Can you work these out from the model? Positions are in its coordinate system, mm. A direction names the side the tool comes from. Give positions to 0.01 mm unless a question says otherwise; leave off trailing zeros. Write each loop counter-clockwise with the first axis right and the second up, starting at its lowest first coordinate (ties: lowest second). Pieces come first, ordered by that corner, then holes.
from build123d import *

# Parameters (mm, degrees)
F0_W     = 2.7374038473
F0_H     = 4.5464726281
F1_DEPTH = 3


with BuildPart() as f1:
    # F0 (on Front) → F1 (new body)
    with BuildSketch(Plane.XZ):
        with BuildLine():
            Line((-13.9879264009, 8.4983842463), (-10.7078288449, 8.4983842463))
            ThreePointArc((-10.7078288449, 8.4983842463), (-12.3096819162, -5.9457433928), (0, -13.6704108706))
            Line((0, -13.6704108706), (29.832560569, -13.6704108706))
            ThreePointArc((29.832560569, -13.6704108706), (41.0439649972, -7.8220549805), (42.6626390029, 4.7190275219))
            ThreePointArc((42.6626390029, 4.7190275219), (52.7277631814, 0.6811115523), (57.2114773095, -9.193492122))
            Line((57.2114773095, -9.193492122), (57.2114773095, 27.5829305145))
            ThreePointArc((57.2114773095, 27.5829305145), (52.7277631814, 17.7083268402), (42.6626390029, 13.6704108706))
            Line((42.6626390029, 13.6704108706), (29.832560569, 13.6704108706))
            Line((29.832560569, 13.6704108706), (0, 13.6704108706))
            Line((0, 13.6704108706), (-14.4307379611, 13.6704108706))
            Line((-14.4307379611, 13.6704108706), (-14.8297163701, 14.5122008398))
            Line((-14.8297163701, 14.5122008398), (-15.268201828, 14.5122008398))
            ThreePointArc((-15.268201828, 14.5122008398), (-15.9753086092, 14.219307621), (-16.268201828, 13.5122008398))
            Line((-16.268201828, 13.5122008398), (-16.268201828, 9.0994058373))
            ThreePointArc((-16.268201828, 9.0994058373), (-15.9753086092, 8.3922990562), (-15.268201828, 8.0994058373))
            Line((-15.268201828, 8.0994058373), (-14.8297163701, 8.0994058373))
            Line((-14.8297163701, 8.0994058373), (-13.9879264009, 8.4983842463))
        make_face()
        with Locations((-10.5523099191, -3.12910098)):
            Rectangle(F0_W, F0_H, mode=Mode.SUBTRACT)
        Polygon((9.3416453156, -8.6632125312), (7.1077647943, -8.6632125312), (4.7967138551, -2.7617063542), (-2.6400774802, -2.7617063542), (-4.9226972128, -8.6632125312), (-7.1078385226, -8.6632125312), (0.2274127889, 9.9714126168), (2.0429484125, 9.9714126168), align=None, mode=Mode.SUBTRACT)
        with Locations((-10.5523099191, 3.0826488801)):
            Rectangle(F0_W, F0_H, mode=Mode.SUBTRACT)
        with BuildLine():
            Line((11.8923307107, -8.6632125312), (11.8923307107, 9.8942421988))
            Line((11.8923307107, 9.8942421988), (17.1358575342, 9.8942421988))
            add(Edge.make_bspline(
                [(17.1358575342, 9.8942421988), (20.8278527957, 9.8942421988), (22.4788935809, 8.7894867411)],
                knots=[0, 0, 0, 1, 1, 1], degree=2))
            add(Edge.make_bspline(
                [(22.4788935809, 8.7894867411), (24.1299343662, 7.6847312833), (24.1299343662, 5.300571527)],
                knots=[0, 0, 0, 1, 1, 1], degree=2))
            add(Edge.make_bspline(
                [(24.1299343662, 5.300571527), (24.1299343662, 3.6474999413), (23.2099817515, 2.5752372911)],
                knots=[0, 0, 0, 1, 1, 1], degree=2))
            add(Edge.make_bspline(
                [(23.2099817515, 2.5752372911), (22.2900291369, 1.5029746409), (20.5232327246, 1.1861697669)],
                knots=[0, 0, 0, 1, 1, 1], degree=2))
            Line((20.5232327246, 1.1861697669), (20.5232327246, 1.0602601376))
            add(Edge.make_bspline(
                [(20.5232327246, 1.0602601376), (24.7513593112, 0.3372951689), (24.7513593112, -3.3831312992)],
                knots=[0, 0, 0, 1, 1, 1], degree=2))
            add(Edge.make_bspline(
                [(24.7513593112, -3.3831312992), (24.7513593112, -5.8688310792), (23.0698565188, -7.2660218052)],
                knots=[0, 0, 0, 1, 1, 1], degree=2))
            add(Edge.make_bspline(
                [(23.0698565188, -7.2660218052), (21.3883537265, -8.6632125312), (18.3665226214, -8.6632125312)],
                knots=[0, 0, 0, 1, 1, 1], degree=2))
            Line((18.3665226214, -8.6632125312), (11.8923307107, -8.6632125312))
        make_face(mode=Mode.SUBTRACT)
        with BuildLine():
            add(Edge.make_bspline(
                [(38.1099648282, -0.6293658567), (39.2065970841, -1.8234765353), (39.2065970841, -3.7243057788)],
                knots=[0, 0, 0, 1, 1, 1], degree=2))
            add(Edge.make_bspline(
                [(39.2065970841, -3.7243057788), (39.2065970841, -6.1734511503), (37.4296466694, -7.5462722706)],
                knots=[0, 0, 0, 1, 1, 1], degree=2))
            add(Edge.make_bspline(
                [(37.4296466694, -7.5462722706), (35.6526962548, -8.919093391), (32.606495544, -8.919093391)],
                knots=[0, 0, 0, 1, 1, 1], degree=2))
            add(Edge.make_bspline(
                [(32.606495544, -8.919093391), (29.3084755745, -8.919093391), (27.5294943594, -8.0661571919)],
                knots=[0, 0, 0, 1, 1, 1], degree=2))
            Line((27.5294943594, -8.0661571919), (27.5294943594, -5.9866175067))
            add(Edge.make_bspline(
                [(27.5294943594, -5.9866175067), (28.6748658267, -6.4658864185), (30.0192557403, -6.7461368839)],
                knots=[0, 0, 0, 1, 1, 1], degree=2))
            add(Edge.make_bspline(
                [(30.0192557403, -6.7461368839), (31.363645654, -7.0263873493), (32.683665962, -7.0263873493)],
                knots=[0, 0, 0, 1, 1, 1], degree=2))
            add(Edge.make_bspline(
                [(32.683665962, -7.0263873493), (34.8403760653, -7.0263873493), (35.9329467202, -6.2079747584)],
                knots=[0, 0, 0, 1, 1, 1], degree=2))
            add(Edge.make_bspline(
                [(35.9329467202, -6.2079747584), (37.0255173751, -5.3895621674), (37.0255173751, -3.9273858262)],
                knots=[0, 0, 0, 1, 1, 1], degree=2))
            add(Edge.make_bspline(
                [(37.0255173751, -3.9273858262), (37.0255173751, -2.9647864016), (36.6376344846, -2.349453858)],
                knots=[0, 0, 0, 1, 1, 1], degree=2))
            add(Edge.make_bspline(
                [(36.6376344846, -2.349453858), (36.2497515941, -1.7341213145), (35.3419837823, -1.2122055927)],
                knots=[0, 0, 0, 1, 1, 1], degree=2))
            add(Edge.make_bspline(
                [(35.3419837823, -1.2122055927), (34.4342159705, -0.6902898709), (32.5821259383, -0.0323105174)],
                knots=[0, 0, 0, 1, 1, 1], degree=2))
            add(Edge.make_bspline(
                [(32.5821259383, -0.0323105174), (29.9948861347, 0.8937344987), (28.8840382755, 2.1629847949)],
                knots=[0, 0, 0, 1, 1, 1], degree=2))
            add(Edge.make_bspline(
                [(28.8840382755, 2.1629847949), (27.7731904163, 3.432235091), (27.7731904163, 5.4752203677)],
                knots=[0, 0, 0, 1, 1, 1], degree=2))
            add(Edge.make_bspline(
                [(27.7731904163, 5.4752203677), (27.7731904163, 7.6197456681), (29.383615192, 8.8889959643)],
                knots=[0, 0, 0, 1, 1, 1], degree=2))
            add(Edge.make_bspline(
                [(29.383615192, 8.8889959643), (30.9940399678, 10.1582462604), (33.6503269876, 10.1582462604)],
                knots=[0, 0, 0, 1, 1, 1], degree=2))
            add(Edge.make_bspline(
                [(33.6503269876, 10.1582462604), (36.416277233, 10.1582462604), (38.7395129751, 9.1428460235)],
                knots=[0, 0, 0, 1, 1, 1], degree=2))
            Line((38.7395129751, 9.1428460235), (38.0652872178, 7.2663863857))
            add(Edge.make_bspline(
                [(38.0652872178, 7.2663863857), (35.7664210814, 8.2289858103), (33.5975261753, 8.2289858103)],
                knots=[0, 0, 0, 1, 1, 1], degree=2))
            add(Edge.make_bspline(
                [(33.5975261753, 8.2289858103), (31.8835305753, 8.2289858103), (30.9189003503, 7.4938360387)],
                knots=[0, 0, 0, 1, 1, 1], degree=2))
            add(Edge.make_bspline(
                [(30.9189003503, 7.4938360387), (29.9542701252, 6.7586862672), (29.9542701252, 5.450850762)],
                knots=[0, 0, 0, 1, 1, 1], degree=2))
            add(Edge.make_bspline(
                [(29.9542701252, 5.450850762), (29.9542701252, 4.4882513374), (30.3096602081, 3.8708879934)],
                knots=[0, 0, 0, 1, 1, 1], degree=2))
            add(Edge.make_bspline(
                [(30.3096602081, 3.8708879934), (30.665050291, 3.2535246493), (31.5098632882, 2.7397321294)],
                knots=[0, 0, 0, 1, 1, 1], degree=2))
            add(Edge.make_bspline(
                [(31.5098632882, 2.7397321294), (32.3546762853, 2.2259396096), (34.0930414909, 1.6045146646)],
                knots=[0, 0, 0, 1, 1, 1], degree=2))
            add(Edge.make_bspline(
                [(34.0930414909, 1.6045146646), (37.0133325723, 0.5647448219), (38.1099648282, -0.6293658567)],
                knots=[0, 0, 0, 1, 1, 1], degree=2))
        make_face(mode=Mode.SUBTRACT)
    extrude(amount=F1_DEPTH)


solid = f1.part
(1) Imagine slicing it at B-B, the plane y = -2.2. Give the number of separate pieces and of enclosed holes in the cut face, plus the area to 3 significant figures.
Returned:
separate pieces: 1
enclosed holes: 5
area: 1,270 mm2
(2) Imagine slicing it at A-A, the plane x = 6. Write out the boundary of the cut face in (y, z), plus the area to 3 significant figures.
Returned:
outline: (-3, -13.67) - (0, -13.67) - (0, -5.83) - (-3, -5.83) - close; (-3, -0.13) - (0, -0.13) - (0, 13.67) - (-3, 13.67) - close
area: 64.9 mm2
(3) Imagine slicing it at C-C, the plane z = 23. Write out the boundary of the cut face in (x, y).
Returned:
outline: (56.25, -3) - (57.21, -3) - (57.21, 0) - (56.25, 0) - close
(4) If I drill on L1, parallel to X at y = -0.4, z = -2.5; L2, parallel to Z at x = 12.5, y = -0.35; L3, parallel to Z at x = 23, y = -0.45, over which ranges is the centre line in solid material (lowest first)?
Returned:
L1: x = -13.44 to -11.92, -9.18 to -4.68, 6.93 to 11.89, 24.69 to 36.72, 39.08 to 43.27, 55.24 to 57.21
L2: z = -13.67 to -8.66, 9.89 to 13.67
L3: z = -13.67 to -7.32, 0.16 to 2.35, 8.37 to 13.67
(5) For faces 1 (the face through (20, -3, 12)), 2 (the face through (-11, -1, 0.809)), which set-ups out of +Z, -Z, +X, -X, +Y, -Y let a thin tool reach every point of the face, with its end or its side?
Returned:
face 1: +Z, -Z, +X, -X, -Y
face 2: +Y, -Y
(6) Will these pins go through, and if not, where does the flat tip stop? P1, Ø1.4, axis at x = -10.5, y = -2, coming from the -Z side; P2, Ø0.9, axis at x = 28, y = -1.5, coming from the +Z side; P3, Ø1.5, axis at y = -2, z = -2, coming from the -X side.
Returned:
P1: stops at z = -9.53
P2: stops at z = 13.67
P3: stops at x = -13.61
(7) If we mould it in two halves opening along Z, with no side actions, what happens to faces 3 (the face through (57.211, -1, 9)), 4 (the face through (-11, -1, -0.856)), 5 (the face through (-11, -1, 5.356)), 6 (the face through (15, -1, 13.67))? For each: +Z half, -Z half, draft (parallel to the pull), parting line (faces both ways), or undercut.
Returned:
face 3: draft
face 4: undercut
face 5: undercut
face 6: +Z half
